Design review of the part built by this model. Coordinates are the model's own, in mm. Face numbers are marked on the shaded views. A direction names the side the tool comes from. Coordinates: 2 decimals unless noted, no trailing zeros. Loops run counter-clockwise (first coordinate to the right, second up) from the corner with the lowest first, then second, coordinate; pieces in that order, holes last. Notation, with made-up numbers: (74, 23) - (105, 23) arc R18 ccw to (105, 53) - close; hole circle Ø4 at (75, 53.5). An arc over 180 degrees is marked (long way). Use one line per item in the form item = value. Start each with the question number.
(1) Clearance check with flat-ended pins moving along their axes: pin 1 Ø2 at (y, z) = (-0.5, 28.5) entering from -X; pin 2 Ø2.5 at (x, z) = (12.5, 24) entering from +Y; pin 3 Ø2 at (x, y) = (11.5, -2) entering from +Z. State where each tip first meets the part, or that it passes through.
(2) For L1, parallel to Z at x = 4.25, y = 7.5; L2, parallel to Z at x = 11, y = -2, list the stretches that pass through material, from the lowest coordinate up.
(3) Tool access review of the marked faces 1, 2, 3 and 4: name each direction out of +Z, -Z, +X, -X, +Y, -Y from which nothing blocks a thin tool from reaching the whole face with its end or side.
(4) Add section A-A (y = 6.75). State the section outline as (x, z) points, plus the area to 3 significant figures.
(5) Add section D-D (y = 3). State the section outline as (x, z) points, plus the area to 3 significant figures.
(6) The part is to be moulded in two halves that separate along Z. For the marked faces 5, 6 and 7, say which applies: pulls with the +Z half, pulls with the -Z half, needs draft (parallel to the pull), parting line crosses it, or undercut.
(7) Add section C-C (x = 14.5). Count the separate pieces of the cut face and the enclosed holes in it, plus the area to 3 significant figures.
(8) Add section B-B (z = 10.5). State the section outline as (x, y) points (3 decimals), plus the area to 3 significant figures.
```python
from build123d import *

# Parameters (mm, degrees)
F1_DEPTH = 38.1
F2_W     = 20.32
F2_H     = 4.699
F3_DEPTH = 5.08
F4_SIZE  = 1.27
F5_SIZE  = 0.635
F6_W     = 3.140959
F6_H     = 6.35
F6_H_2   = 13.208
F6_H_3   = 5.842
F7_DEPTH = 19.051
F8_SIZE  = 0.635


with BuildPart() as f1:
    # F0 (on Top) → F1 (new body)
    with BuildSketch(Plane.XY):
        Polygon((-1.27, 6.223), (0, 4.953), (17.78, 4.953), (19.05, 6.223), (19.05, 7.493), (17.78, 8.763), (8.89, 8.763), (0, 8.763), (-1.27, 7.493), align=None)
        Polygon((17.78, 4.953), (0, 4.953), (0, 0), (4.445, 0), (4.445, -1.27), (2.794, -1.27), (2.794, -3.140959), (8.89, -3.140959), (14.986, -3.140959), (14.986, -1.27), (13.335, -1.27), (13.335, 0), (17.78, 0), align=None)
    extrude(amount=F1_DEPTH)

    # F2 (on face) → F3 (cut)
    with BuildSketch(Plane(origin=(0, 8.763, 0), x_dir=(-1, 0, 0), z_dir=(0, 1, 0))):
        with Locations((-8.89, 34.0995)):
            Rectangle(F2_W, F2_H)
        with Locations((-8.89, 24.0665)):
            Rectangle(F2_W, F2_H)
        with Locations((-8.89, 14.0335)):
            Rectangle(F2_W, F2_H)
        with Locations((-8.89, 4.0005)):
            Rectangle(F2_W, F2_H)
    extrude(amount=-F3_DEPTH, mode=Mode.SUBTRACT)

    # F4
    f4_edges = [f1.edges().sort_by_distance(p)[0] for p in [
        (8.89, 3.683, 36.449),
        (8.89, 3.683, 31.75),
        (8.89, 3.683, 26.416),
        (8.89, 3.683, 21.717),
        (8.89, 3.683, 16.383),
        (8.89, 3.683, 11.684),
        (8.89, 3.683, 6.35),
        (8.89, 3.683, 1.651),
    ]]
    chamfer(f4_edges, length=F4_SIZE)

    # F5
    f5_edges = [f1.edges().sort_by_distance(p)[0] for p in [
        (8.89, 8.763, 31.75),
        (8.89, 8.763, 26.416),
        (8.89, 8.763, 21.717),
        (8.89, 8.763, 16.383),
        (8.89, 8.763, 11.684),
        (8.89, 8.763, 6.35),
        (8.89, 8.763, 1.651),
        (8.89, 8.763, 36.449),
    ]]
    chamfer(f5_edges, length=F5_SIZE)

    # F6 (on face) → F7 (cut, through all)
    with BuildSketch(Plane.YZ.offset(17.78)):
        with Locations((-1.57048, 34.925)):
            Rectangle(F6_W, F6_H)
        with Locations((-1.57048, 18.796)):
            Rectangle(F6_W, F6_H_2)
        with Locations((-1.57048, 2.921)):
            Rectangle(F6_W, F6_H_3)
    extrude(amount=-F7_DEPTH, mode=Mode.SUBTRACT)

    # F8
    f8_edges = [f1.edges().sort_by_distance(p)[0] for p in [
        (8.89, -3.140959, 31.75),
        (8.89, -3.140959, 12.192),
        (8.89, -3.140959, 25.4),
        (8.89, -3.140959, 5.842),
    ]]
    chamfer(f8_edges, length=F8_SIZE)


solid = f1.part
```
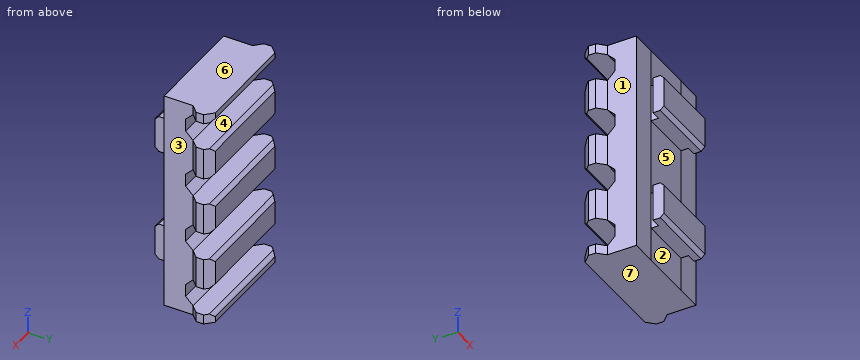
Computed values:
q1.pin_1 = 0
q1.pin_2 = 3.92
q1.pin_3 = 31.75
q2.L1 = 0 to 1.65, 6.35 to 11.68, 16.38 to 21.72, 26.42 to 31.75, 36.45 to 38.1
q2.L2 = 5.84 to 12.19, 25.4 to 31.75
q3.face_1 = +Z, -Z, -X, -Y
q3.face_2 = -Z, +X, -X, -Y
q3.face_3 = +Z, -Z, +X, -Y
q3.face_4 = +X, -X, +Y
q4.outline = (-1.27, 0) - (19.05, 0) - (19.05, 1.65) - (-1.27, 1.65) - close; (-1.27, 6.35) - (19.05, 6.35) - (19.05, 11.68) - (-1.27, 11.68) - close; (-1.27, 16.38) - (19.05, 16.38) - (19.05, 21.72) - (-1.27, 21.72) - close; (-1.27, 26.42) - (19.05, 26.42) - (19.05, 31.75) - (-1.27, 31.75) - close; (-1.27, 36.45) - (19.05, 36.45) - (19.05, 38.1) - (-1.27, 38.1) - close
q4.area = 392 mm^2
q5.outline = (0, 0) - (17.78, 0) - (17.78, 38.1) - (0, 38.1) - close
q5.area = 677 mm^2
q6.face_5 = undercut
q6.face_6 = pulls with the +Z half
q6.face_7 = pulls with the -Z half
q7.separate_pieces = 3
q7.enclosed_holes = 0
q7.area = 266 mm^2
q8.outline = (-1.27, 6.223) - (0, 4.953) - (0, 0) - (4.445, 0) - (4.445, -1.27) - (2.794, -1.27) - (2.794, -3.141) - (14.986, -3.141) - (14.986, -1.27) - (13.335, -1.27) - (13.335, 0) - (17.78, 0) - (17.78, 4.953) - (19.05, 6.223) - (19.05, 7.493) - (17.78, 8.763) - (0, 8.763) - (-1.27, 7.493) - close
q8.area = 196 mm^2
